Model file for the job. Use its own axes, mm. A direction names the side the tool comes from. Round coordinates to 2 decimals unless told otherwise and drop trailing zeros. Order: outer loops, then holes, each group sorted by start corner. A loop starts at its lowest first (then second) coordinate and runs counter-clockwise, first axis right, second up. Notation, with made-up numbers: (44, -30) - (54, -30) arc R11 cw to (54, -11) - close; hole circle Ø1 at (-6.75, 31). An arc over 180 degrees is marked (long way). Put each result on its own line as item: value. Start each with the question number.
Item 1: Saw through at B-B on x = -25. List the corners of the cut face in (y, z), plus the area to 3 significant figures.
Item 2: Pin check, flat tips, straight feed: pin 1 Ø5 at (y, z) = (8, 3) entering from -X; pin 2 Ø6 at (y, z) = (-1, 2.5) entering from -X; pin 3 Ø3 at (y, z) = (-2, 5.5) entering from +X; pin 4 Ø3.5 at (x, z) = (25, 5) entering from +Y (1 decimal). Stop position of each tip, or through.
Item 3: Which spindle directions (+Z, -Z, +X, -X, +Y, -Y) get a long thin tool onto all of the face, cutting with end or side? Do faces 4 (the face through (22, -15, 5)), 5 (the face through (18, -20, 5)), 6 (the face through (5, -18, 5)). Say none if no direction does.
Item 4: Probe probe 1 along Z at (x, y) = (25, -16); probe 2 along X at (y, z) = (-17.5, 7.75); probe 3 along X at (y, z) = (0, 4.5) (3 decimals). List the from-to ranges inside material, lowest first.
Item 5: Mould opens along Y. For faces 1 (the face through (-5, -18, 5)), 2 (the face through (-0.627, 15.863, 4.93)), 3 (the face through (-17, -20, 5)) say: pulls with the +Y half, pulls with the -Y half, needs draft (parallel to the pull), parting line crosses it, or undercut.
Item 6: Saw through at A-A on z = 5. List the corners of the cut face in (x, y) (3 decimals), plus the area to 3 significant figures.
Item 7: Saw through at D-D on z = 8. List the corners of the cut face in (x, y) (3 decimals), plus the area to 3 significant figures.
Item 8: Saw through at C-C on y = 0. List the corners of the cut face in (x, z) (3 decimals).
```python
from build123d import *

# Parameters (mm, degrees)
SKETCH1_R             = 20
BOSS_EXTRUDE1_DEPTH   = 10
SKETCH2_W             = 60
SKETCH2_H             = 5
BOSS_EXTRUDE2_DEPTH   = 10
SKETCH3_R             = 15.875
CUT_EXTRUDE1_DEPTH    = 38.416573868
SKETCH4_W             = 10
SKETCH4_H             = 4.932962302
CUT_EXTRUDE2_DEPTH    = 38.416573868
F_6_CLEARANCE_HOLE1_D = 3.7973


with BuildPart() as part:
    # Sketch1 → Boss-Extrude1 (new body)
    with BuildSketch(Plane.XY):
        Circle(SKETCH1_R)
    extrude(amount=BOSS_EXTRUDE1_DEPTH)

    # Sketch2 → Boss-Extrude2 (add)
    with BuildSketch(Plane(origin=(0, 0, 0), x_dir=(-1, 0, 0), z_dir=(0, 0, -1))):
        with Locations((0, -17.5)):
            Rectangle(SKETCH2_W, SKETCH2_H)
    extrude(amount=-BOSS_EXTRUDE2_DEPTH)

    # Sketch3 → Cut-Extrude1 (cut, through all)
    with BuildSketch(Plane(origin=(0, 0, 0), x_dir=(-1, 0, 0), z_dir=(0, 0, -1))):
        Circle(SKETCH3_R)
    extrude(amount=-CUT_EXTRUDE1_DEPTH, mode=Mode.SUBTRACT)

    # Sketch4 → Cut-Extrude2 (cut, through all)
    with BuildSketch(Plane.XY.offset(10)):
        with Locations((0, -17.533518849)):
            Rectangle(SKETCH4_W, SKETCH4_H)
    extrude(amount=-CUT_EXTRUDE2_DEPTH, mode=Mode.SUBTRACT)

    # #6 Clearance Hole1 (through all)
    with Locations(Plane(origin=(0, -15, 0), x_dir=(1, 0, 0), z_dir=(0, 1, 0))):
        with Locations((-25, -5)):
            f_6_clearance_hole1 = Hole(F_6_CLEARANCE_HOLE1_D / 2)

    # Mirror1: #6 Clearance Hole1 across plane
    add(f_6_clearance_hole1.mirror(Plane(origin=(0, 0, 0), x_dir=(0, 0, 1), z_dir=(1, 0, 0))), mode=Mode.SUBTRACT)


solid = part.part
```
Results found:
1. outline: (-20, 0) - (-15, 0) - (-15, 3.1) - (-20, 3.1) - close; (-20, 6.9) - (-15, 6.9) - (-15, 10) - (-20, 10) - close
1. area: 31.0 mm²
2. pin 1: stops at x = -19.23
2. pin 2: stops at x = -20
2. pin 3: stops at x = 19.99
2. pin 4: passes through
3. face 4: +Z, -Z, +X
3. face 5: +Z, -Z, +X, -X, -Y
3. face 6: +Z, -Z, -Y
4. probe 1: z = 0 to 3.1, 6.9 to 10
4. probe 2: x = -30 to -5, 5 to 30
4. probe 3: x = -20 to -15.875, 15.875 to 20
5. face 1: needs draft
5. face 2: undercut
5. face 3: pulls with the -Y half
6. outline: (-30, -20) - (-26.899, -20) - (-26.899, -15) - (-30, -15) - close; (-23.101, -20) - (-5, -20) - (-5, -15.067) arc R15.875 cw (long way) to (5, -15.067) - (5, -20) - (23.101, -20) - (23.101, -15) - (13.229, -15) arc R20 ccw (long way) to (-13.229, -15) - (-23.101, -15) - close; (26.899, -20) - (30, -20) - (30, -15) - (26.899, -15) - close
6. area: 592 mm²
7. outline: (-30, -20) - (-5, -20) - (-5, -15.067) arc R15.875 cw (long way) to (5, -15.067) - (5, -20) - (30, -20) - (30, -15) - (13.229, -15) arc R20 ccw (long way) to (-13.229, -15) - (-30, -15) - close
7. area: 630 mm²
8. outline: (-20, 0) - (-15.875, 0) - (-15.875, 10) - (-20, 10) - close; (15.875, 0) - (20, 0) - (20, 10) - (15.875, 10) - close
